Build history of the part. All positions in model axes, mm. A direction names the side the tool comes from. Give positions to 0.01 mm unless a question says otherwise; leave off trailing zeros. Order: outer loops, then holes, each group sorted by start corner. A loop starts at its lowest first (then second) coordinate and runs counter-clockwise, first axis right, second up. Notation, with made-up numbers: (73.25, 87) - (106.25, 87) arc R15 ccw to (106.25, 92) - close; hole circle Ø7 at (70.25, 84.25). An arc over 180 degrees is marked (long way). Answer in a Markdown table with one row per item.
```python
from build123d import *

# Parameters (mm, degrees)
SKETCH1_R           = 11
BOSS_EXTRUDE1_DEPTH = 10
SKETCH1_3_W         = 50
SKETCH1_3_H         = 10
BOSS_EXTRUDE2_DEPTH = 25
SKETCH1_4_R         = 11
SKETCH1_4_R_2       = 4
BOSS_EXTRUDE3_DEPTH = 19


with BuildPart() as part:
    # Sketch1 → Boss-Extrude1 (new body)
    with BuildSketch(Plane.XY):
        with BuildLine():
            Line((-25, -3.685481934), (-25, -32))
            Line((-25, -32), (25, -32))
            Line((25, -32), (25, -3.685481934))
            ThreePointArc((25, -3.685481934), (28.70821268, 15.210825292), (39.28281707, 31.304271474))
            ThreePointArc((39.28281707, 31.304271474), (42.127486852, 38.789799017), (38.567256581, 45.962666587))
            ThreePointArc((38.567256581, 45.962666587), (0, 60), (-38.567256581, 45.962666587))
            ThreePointArc((-38.567256581, 45.962666587), (-42.127486852, 38.789799017), (-39.28281707, 31.304271474))
            ThreePointArc((-39.28281707, 31.304271474), (-28.70821268, 15.210825292), (-25, -3.685481934))
        make_face()
        Circle(SKETCH1_R, mode=Mode.SUBTRACT)
        with BuildLine():
            ThreePointArc((-28.925442436, 34.47199994), (-35.9696027, 35.088284108), (-35.353318533, 42.132444372))
            ThreePointArc((-35.353318533, 42.132444372), (0, 55), (35.353318533, 42.132444372))
            ThreePointArc((35.353318533, 42.132444372), (35.9696027, 35.088284108), (28.925442436, 34.47199994))
            ThreePointArc((28.925442436, 34.47199994), (0, 45), (-28.925442436, 34.47199994))
        make_face(mode=Mode.SUBTRACT)
    extrude(amount=BOSS_EXTRUDE1_DEPTH)

    # Sketch1<3> → Boss-Extrude2 (add)
    with BuildSketch(Plane.XY):
        with Locations((0, -37)):
            Rectangle(SKETCH1_3_W, SKETCH1_3_H)
    extrude(amount=BOSS_EXTRUDE2_DEPTH)

    # Sketch1<4> → Boss-Extrude3 (add)
    with BuildSketch(Plane.XY):
        Circle(SKETCH1_4_R)
        Circle(SKETCH1_4_R_2, mode=Mode.SUBTRACT)
    extrude(amount=BOSS_EXTRUDE3_DEPTH)


solid = part.part
```
1. Cut at B-B on x = -18.5. Write the cut outline in (y, z).
Check result:
| item | result |
|---|---|
| outline | (-42, 0) - (41.02, 0) - (41.02, 10) - (-32, 10) - (-32, 25) - (-42, 25) - close; (51.8, 0) - (57.08, 0) - (57.08, 10) - (51.8, 10) - close |
2. Cut at D-D on y = 2. Write the cut outline in (x, z).
Check result:
| item | result |
|---|---|
| outline | (-25.32, 0) - (-3.46, 0) - (-3.46, 19) - (-10.82, 19) - (-10.82, 10) - (-25.32, 10) - close; (3.46, 0) - (25.32, 0) - (25.32, 10) - (10.82, 10) - (10.82, 19) - (3.46, 19) - close |
3. Cut at A-A on z = 12.5. Write the cut outline in (x, y).
Check result:
| item | result |
|---|---|
| outline | (-25, -42) - (25, -42) - (25, -32) - (-25, -32) - close; circle Ø22 at (0, 0); hole circle Ø8 at (0, 0) |
4. Drop flat-ended pins along their axis: P1, Ø12.5, axis at y = -26, z = 17.5, coming from the -X side; P2, Ø24, axis at x = -3.5, y = 3, coming from the +Z side; P3, Ø4, axis at x = -2, z = 7.5, coming from the +Y side; P4, Ø12, axis at x = -15.5, y = -18.5, coming from the -Z side. Give the stop position or say it passes through.
Check result:
| item | result |
|---|---|
| P1 | stops at x = -25 |
| P2 | stops at z = 19 |
| P3 | stops at y = 60 |
| P4 | stops at z = 0 |
5. Which spindle directions (+Z, -Z, +X, -X, +Y, -Y) get a long thin tool onto all of the face, cutting with end or side? Do faces 4 (the face through (0, -32, 17)), 5 (the face through (-2.38, -10.74, 14.44)), 6 (the face through (25, -27, 7)), 7 (the face through (-0.538, 54.997, 4.93)). Say none if no direction does.
Check result:
| item | result |
|---|---|
| face 4 | +Z, +X, -X |
| face 5 | +Z |
| face 6 | +Z, -Z, +X, -Y |
| face 7 | +Z, -Z |
6. Two-plate mould, pull along Y, no slides. Class faces 1 (the face through (0, -42, 12)), 2 (the face through (42.132, 38.675, 4.93)), 3 (the face through (0, 45, 5)): +Y half, -Y half, draft (parallel to the pull), parting line (faces both ways), or undercut.
Check result:
| item | result |
|---|---|
| face 1 | -Y half |
| face 2 | parting line |
| face 3 | undercut |
7. Cut at C-C on z = 5.5. Write the cut outline in (x, y), and give its area (3 significant figures).
Check result:
| item | result |
|---|---|
| outline | (-39.28, 31.3) arc R50 cw to (-25, -3.69) - (-25, -42) - (25, -42) - (25, -3.69) arc R50 cw to (39.28, 31.3) arc R10 ccw to (38.57, 45.96) arc R60 ccw to (-38.57, 45.96) arc R10 ccw to start; hole (-35.35, 42.13) arc R5 ccw to (-28.93, 34.47) arc R45 cw to (28.93, 34.47) arc R5 ccw to (35.35, 42.13) arc R55 ccw to start; hole circle Ø8 at (0, 0) |
| area | 5,100 mm² |
8. Probe line 1 (Y direction, x = 0, z = 4.25); line 2 (Y direction, x = 0, z = 14.75); line 3 (Z direction, x = -6, y = -14). List the from-to ranges inside material, lowest first.
Check result:
| item | result |
|---|---|
| line 1 | y = -42 to -4, 4 to 45, 55 to 60 |
| line 2 | y = -42 to -32, -11 to -4, 4 to 11 |
| line 3 | z = 0 to 10 |
